```python
from build123d import *

# Parameters (mm, degrees)
SKETCH1_R            = 6
BOSS_EXTRUDE1_DEPTH  = 12.5
SKETCH2_W            = 30
SKETCH2_H            = 50
SKETCH2_R            = 7.5
BOSS_EXTRUDE2_DEPTH  = 12.5
FILLET1_R            = 15
FILLET1_OF_MIRROR1_R = 15


with BuildPart() as part:
    # Sketch1 → Boss-Extrude1 (new body)
    with BuildSketch(Plane(origin=(0, 0, 0), x_dir=(1, 0, 0), z_dir=(0, 1, 0))):
        with BuildLine():
            Line((-45.931122004, 12.73174394), (-15, 32))
            Line((-15, 32), (15, 32))
            Line((15, 32), (45.931122004, 12.73174394))
            ThreePointArc((45.931122004, 12.73174394), (53, 0), (45.931122004, -12.73174394))
            Line((45.931122004, -12.73174394), (15, -32))
            Line((15, -32), (-15, -32))
            Line((-15, -32), (-45.931122004, -12.73174394))
            ThreePointArc((-45.931122004, -12.73174394), (-53, 0), (-45.931122004, 12.73174394))
        make_face()
        with Locations(Location((-38, 0, 0), (0, 0, 270))):
            Circle(SKETCH1_R, mode=Mode.SUBTRACT)
        with Locations(Location((38, 0, 0), (0, 0, 90))):
            Circle(SKETCH1_R, mode=Mode.SUBTRACT)
    extrude(amount=BOSS_EXTRUDE1_DEPTH)

    # Sketch2 → Boss-Extrude2 (add)
    with BuildSketch(Plane.XY.offset(32)):
        with Locations((0, 25)):
            Rectangle(SKETCH2_W, SKETCH2_H)
        with Locations((0, 35)):
            Circle(SKETCH2_R, mode=Mode.SUBTRACT)
    boss_extrude2 = extrude(amount=-BOSS_EXTRUDE2_DEPTH)

    # Fillet1
    fillet1_edges = [part.edges().sort_by_distance(p)[0] for p in [
        (15, 50, 25.75),
        (-15, 50, 25.75),
    ]]
    fillet(fillet1_edges, radius=FILLET1_R - 0.0001)  # a hair under: the kernel refuses the full size

    # Mirror1: Boss-Extrude2 across plane
    add(boss_extrude2.mirror(Plane.XY))

    # Fillet1 of Mirror1
    fillet1_of_mirror1_edges = [part.edges().sort_by_distance(p)[0] for p in [
        (15, 50, -25.75),
        (-15, 50, -25.75),
    ]]
    fillet(fillet1_of_mirror1_edges, radius=FILLET1_OF_MIRROR1_R - 0.0001)  # a hair under: the kernel refuses the full size


solid = part.part
```
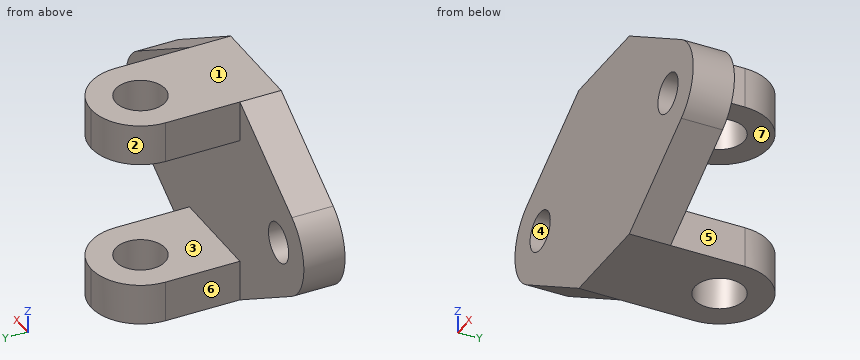
Check sheet for the modelled part. Datum: model origin and axes. Units: mm. Face numbers are marked on the shaded views. A direction names the side the tool comes from. Give positions to 0.01 mm unless a question says otherwise; leave off trailing zeros. Write each loop counter-clockwise with the first axis right and the second up, starting at its lowest first coordinate (ties: lowest second). Pieces come first, ordered by that corner, then holes.
Item 1: Scan lines: L1, parallel to Y at x = -28, z = -22; L2, parallel to X at y = 31, z = -21; L3, parallel to Z at x = 38, y = 3. Record each from-to range of solid material in increasing order.
Item 2: Draft check along Z on the marked faces 1, 2 and 3. Enter one of: released by +Z, released by -Z, zero draft, split by the parting line, or undercut.
Item 3: Cross-section at B-B (z = 0). Enter the section's corners in (x, y).
Item 4: Access from +Z, -Z, +X, -X, +Y, -Y to the whole of each face (thin tool, end or side, straight path). Record for the marked faces 4, 5, 6 and 7.
Item 5: Cross-section at C-C (x = 38). Enter the section's corners in (y, z).
Item 6: Cross-section at A-A (y = 17). Enter the section's corners in (x, z).
Item 7: Gauge pin test, flat ends, axial feed: pin 1 (2 mm diameter, centred on x = 15, z = 14, fed in from +Y); pin 2 (10 mm diameter, centred on y = 19.5, z = 24.5, fed in from -X); pin 3 (14 mm diameter, centred on y = 20.5, z = -25, fed in from +X). Record the tip position at first contact, or that the pin passes through.
Report:
1. L1: y = 0 to 12.5
1. L2: x = -15 to -6.34, 6.34 to 15
1. L3: z = -17.67 to -6, 6 to 17.67
2. face 1: released by +Z
2. face 2: zero draft
2. face 3: undercut
3. outline: (-53, 0) - (-44, 0) - (-44, 12.5) - (-53, 12.5) - close; (-32, 0) - (32, 0) - (32, 12.5) - (-32, 12.5) - close; (44, 0) - (53, 0) - (53, 12.5) - (44, 12.5) - close
4. face 4: +Y, -Y
4. face 5: +Z, -Z, +X, +Y
4. face 6: +Z, -Z, -X, +Y
4. face 7: +X, -X, +Y
5. outline: (0, -17.67) - (12.5, -17.67) - (12.5, -6) - (0, -6) - close; (0, 6) - (12.5, 6) - (12.5, 17.67) - (0, 17.67) - close
6. outline: (-15, -32) - (15, -32) - (15, -19.5) - (-15, -19.5) - close; (-15, 19.5) - (15, 19.5) - (15, 32) - (-15, 32) - close
7. pin 1: stops at y = 12.5
7. pin 2: stops at x = -15
7. pin 3: stops at x = 15
